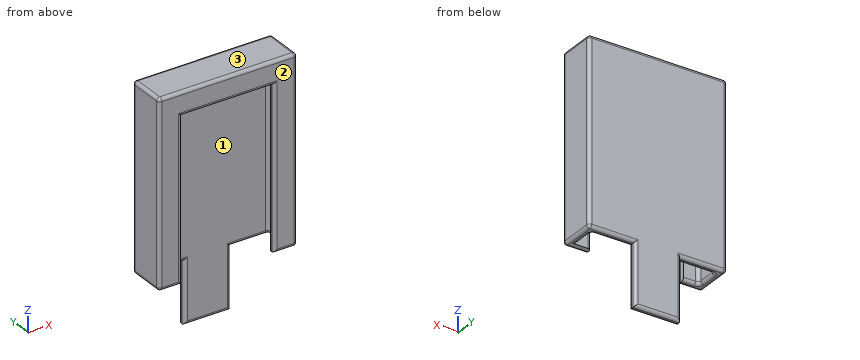
from build123d import *

# Parameters (mm, degrees)
F0_W     = 90
F0_H     = 25
F0_W_2   = 80
F0_H_2   = 15
F1_DEPTH = 120
F3_DEPTH = 110
F2_W     = 60
F2_H     = 105
F4_DEPTH = 10
F5_W     = 30
F5_H     = 40
F6_DEPTH = 5
F7_R     = 2


with BuildPart() as f1:
    # F0 (on Top) → F1 (new body)
    with BuildSketch(Plane.XY):
        Rectangle(F0_W, F0_H)
        Rectangle(F0_W_2, F0_H_2, mode=Mode.SUBTRACT)
        Rectangle(F0_W_2, F0_H_2)
    extrude(amount=F1_DEPTH)

    # F0 (on Top) → F3 (cut)
    with BuildSketch(Plane.XY):
        Rectangle(F0_W_2, F0_H_2)
    extrude(amount=F3_DEPTH, mode=Mode.SUBTRACT)

    # F2 (on face) → F4 (cut)
    with BuildSketch(Plane.XZ.offset(12.5)):
        with Locations((0, 52.5)):
            Rectangle(F2_W, F2_H)
    extrude(amount=-F4_DEPTH, mode=Mode.SUBTRACT)

    # F5 (on face) → F6 (join)
    with BuildSketch(Plane(origin=(0, 12.5, 0), x_dir=(-1, 0, 0), z_dir=(0, 1, 0))):
        with Locations((0, -20)):
            Rectangle(F5_W, F5_H)
    extrude(amount=-F6_DEPTH)

    # F7
    f7_edges = [f1.edges().sort_by_distance(p)[0] for p in [
        (40, 7.5, 55),
        (0, 7.5, 110),
        (-40, 7.5, 55),
        (-27.5, 7.5, 0),
        (-15, 7.5, -20),
        (0, 7.5, -40),
        (15, 7.5, -20),
        (27.5, 7.5, 0),
        (30, -7.5, 52.5),
        (-40, -7.5, 55),
        (-40, 0, 110),
        (0, -7.5, 110),
        (40, 0, 110),
        (-37.5, -12.5, 0),
        (-30, -12.5, 52.5),
        (0, -12.5, 105),
        (30, -12.5, 52.5),
        (37.5, -12.5, 0),
        (45, -12.5, 60),
        (0, -12.5, 120),
        (-45, -12.5, 60),
        (45, 12.5, 60),
        (45, 0, 0),
        (45, 0, 120),
        (0, 12.5, 120),
        (-45, 12.5, 60),
        (-30, 12.5, 0),
        (-15, 12.5, -20),
        (0, 12.5, -40),
        (15, 12.5, -20),
        (30, 12.5, 0),
        (-45, 0, 0),
        (-45, 0, 120),
        (-40, 0, 0),
        (-35, -7.5, 0),
        (40, 0, 0),
    ]]
    fillet(f7_edges, radius=F7_R)


solid = f1.part
Geometry: final body of the model. Coordinates: model frame, mm. Face numbers are marked on the shaded views. Round coordinates to 2 decimals unless told otherwise and drop trailing zeros. Order: outer loops, then holes, each group sorted by start corner. A loop starts at its lowest first (then second) coordinate and runs counter-clockwise, first axis right, second up. Notation, with made-up numbers: (35, -12.75) -> (88, -12.75) arc R14 cw to (88, 8.25) -> close; hole circle Ø1 at (68, -23). An arc over 180 degrees is marked (long way). Put each result on its own line as item: value. Start each with the question number.
Q1. Section A-A on z = -12.5. Return the cut outline in (x, y), and give its area (3 significant figures).
Q2. Pull-direction query (Y, two-part tool) for the marked faces 1, 2 and 3; classes: +Y half, -Y half, draft (parallel to the pull), parting line (faces both ways), or undercut.
Q3. Line query: probe 1 along X at (y, z) = (0.75, 15); probe 2 along Y at (x, z) = (34, 94.5); probe 3 along Y at (x, z) = (-9, -1.5). Output: solid intervals per line, ascending.
Q4. Section C-C on x = 26. Return the cut outline in (y, z), and give its area (3 significant figures).
Q5. Section D-D on z = 31. Return the cut outline in (x, y).
Q6. Section B-B on y = 4. Return the cut outline in (x, z), and give its area (3 significant figures).
Q7. First-contact query: pin 1 (6.5 mm diameter, centred on x = -28.5, y = -4, fed in from -Z); pin 2 (0.9 mm diameter, centred on x = 14, y = -8.5, fed in from -Z); pin 3 (3.5 mm diameter, centred on x = 7.5, y = -1, fed in from -Z). Flat tips, straight axial feed; report the tip coordinate or a pass-through.
Ans:
1. outline: (-15, 9.5) arc R2 ccw to (-13, 7.5) -> (13, 7.5) arc R2 ccw to (15, 9.5) -> (15, 10.5) arc R2 ccw to (13, 12.5) -> (-13, 12.5) arc R2 ccw to (-15, 10.5) -> close
1. area: 147 mm2
2. face 1: undercut
2. face 2: -Y half
2. face 3: draft
3. probe 1: x = -45 to -40, 40 to 45
3. probe 2: y = -12.5 to -7.5, 7.5 to 12.5
3. probe 3: y = 7.5 to 12.5
4. outline: (-12.5, 107) arc R2 ccw to (-10.5, 105) -> (-7.5, 105) -> (-7.5, 108) arc R2 cw to (-5.5, 110) -> (5.5, 110) arc R2 cw to (7.5, 108) -> (7.5, 2) arc R2 ccw to (9.5, 0) -> (10.5, 0) arc R2 ccw to (12.5, 2) -> (12.5, 118) arc R2 ccw to (10.5, 120) -> (-10.5, 120) arc R2 ccw to (-12.5, 118) -> close
4. area: 822 mm2
5. outline: (-45, -10.5) arc R2 ccw to (-43, -12.5) -> (-32, -12.5) arc R2 ccw to (-30, -10.5) -> (-30, -7.5) -> (-38, -7.5) arc R2 cw to (-40, -5.5) -> (-40, 5.5) arc R2 cw to (-38, 7.5) -> (38, 7.5) arc R2 cw to (40, 5.5) -> (40, -7.5) -> (32, -7.5) arc R2 ccw to (30, -9.5) -> (30, -10.5) arc R2 ccw to (32, -12.5) -> (43, -12.5) arc R2 ccw to (45, -10.5) -> (45, 10.5) arc R2 ccw to (43, 12.5) -> (-43, 12.5) arc R2 ccw to (-45, 10.5) -> close
6. outline: (-45, 2) arc R2 ccw to (-43, 0) -> (-42, 0) arc R2 ccw to (-40, 2) -> (-40, 108) arc R2 cw to (-38, 110) -> (38, 110) arc R2 cw to (40, 108) -> (40, 2) arc R2 ccw to (42, 0) -> (43, 0) arc R2 ccw to (45, 2) -> (45, 118) arc R2 ccw to (43, 120) -> (-43, 120) arc R2 ccw to (-45, 118) -> close
6. area: 2,000 mm2
7. pin 1: stops at z = 108.97
7. pin 2: stops at z = 105
7. pin 3: stops at z = 110
